from build123d import *

# Parameters (mm, degrees)
F1_DEPTH    = 12.7
F6_DEPTH    = 25.4
F7_T1_DEPTH = 49.4232912098
F7_T4_ANGLE = 29.8619681209
F7_T6_ANGLE = 29.8619681209
F8_START    = -2.159
F8_DEPTH    = 23.241
F9_DEPTH    = 25.4


# Not quite as in the source:
# - a fillet or chamfer that OpenCascade refuses, or shapes differently, is made with other operations: its cross-section is extruded or revolved along the edge and cut away or added


with BuildPart() as f1:
    # F0 (on Top) → F1 (new body, symmetric)
    with BuildSketch(Plane.XY):
        with BuildLine():
            ThreePointArc((0, 101.6), (-6.6449579298, 101.382466601), (-13.2614611296, 100.7307979156))
            Line((-13.2614611296, 100.7307979156), (-12.6812722051, 96.3238255068))
            ThreePointArc((-12.6812722051, 96.3238255068), (-6.3542410204, 96.9469836872), (0, 97.155))
            Line((0, 97.155), (0, 101.6))
        make_face()
        with BuildLine():
            Line((12.6812722051, 96.3238255068), (13.2614611296, 100.7307979156))
            ThreePointArc((13.2614611296, 100.7307979156), (6.6449579298, 101.382466601), (0, 101.6))
            Line((0, 101.6), (0, 97.155))
            ThreePointArc((0, 97.155), (6.3542410204, 96.9469836872), (12.6812722051, 96.3238255068))
        make_face()
    extrude(amount=F1_DEPTH, both=True)

    # F5 (on line) → F6 (cut)
    with BuildSketch(Plane(origin=(0, 101.6, 0), x_dir=(-1, 0, 0), z_dir=(0, 1, 0))):
        with BuildLine():
            Line((6.35, -6.35), (4.9276, -6.35))
            ThreePointArc((4.9276, -6.35), (6.35, -7.7724), (7.7724, -6.35))
            ThreePointArc((7.7724, -6.35), (7.3557886856, -5.3442113144), (6.35, -4.9276))
            Line((6.35, -4.9276), (6.35, -6.35))
        make_face()
        with BuildLine():
            ThreePointArc((6.35, -4.9276), (5.3442113144, -5.3442113144), (4.9276, -6.35))
            Line((4.9276, -6.35), (6.35, -6.35))
            Line((6.35, -6.35), (6.35, -4.9276))
        make_face()
        with BuildLine():
            Line((-4.9276, -6.35), (-6.35, -6.35))
            Line((-6.35, -6.35), (-6.35, -4.9276))
            ThreePointArc((-6.35, -4.9276), (-7.3557886856, -7.3557886856), (-4.9276, -6.35))
        make_face()
        with BuildLine():
            Line((-6.35, -4.9276), (-6.35, -6.35))
            Line((-6.35, -6.35), (-4.9276, -6.35))
            ThreePointArc((-4.9276, -6.35), (-5.3442113144, -5.3442113144), (-6.35, -4.9276))
        make_face()
        with BuildLine():
            Line((6.35, 6.35), (6.35, 4.9276))
            ThreePointArc((6.35, 4.9276), (7.3557886856, 5.3442113144), (7.7724, 6.35))
            ThreePointArc((7.7724, 6.35), (6.35, 7.7724), (4.9276, 6.35))
            Line((4.9276, 6.35), (6.35, 6.35))
        make_face()
        with BuildLine():
            ThreePointArc((4.9276, 6.35), (5.3442113144, 5.3442113144), (6.35, 4.9276))
            Line((6.35, 4.9276), (6.35, 6.35))
            Line((6.35, 6.35), (4.9276, 6.35))
        make_face()
        with BuildLine():
            ThreePointArc((-4.9276, 6.35), (-7.3557886856, 7.3557886856), (-6.35, 4.9276))
            Line((-6.35, 4.9276), (-6.35, 6.35))
            Line((-6.35, 6.35), (-4.9276, 6.35))
        make_face()
        with BuildLine():
            Line((-6.35, 6.35), (-6.35, 4.9276))
            ThreePointArc((-6.35, 4.9276), (-5.3442113144, 5.3442113144), (-4.9276, 6.35))
            Line((-4.9276, 6.35), (-6.35, 6.35))
        make_face()
    extrude(amount=-F6_DEPTH, mode=Mode.SUBTRACT)

    # F7: fillet of radius 5.08 on 4 edges, made by hand

    # F7_s2 → F7_t1 (cut)
    with BuildSketch(Plane.XY.offset(-24.7116456049)):
        with BuildLine():
            ThreePointArc((7.9036679621, 96.8329802172), (11.3054660928, 97.7882158705), (13.2614611296, 100.7307979156))
            Line((13.2614611296, 100.7307979156), (12.6812722051, 96.3238255068))
            ThreePointArc((12.6812722051, 96.3238255068), (10.2956180024, 96.6079410553), (7.9036679621, 96.8329802172))
        make_face()
        with BuildLine():
            ThreePointArc((-7.9036679621, 96.8329802172), (-11.3054660928, 97.7882158705), (-13.2614611296, 100.7307979156))
            Line((-13.2614611296, 100.7307979156), (-12.6812722051, 96.3238255068))
            ThreePointArc((-12.6812722051, 96.3238255068), (-10.2956180024, 96.6079410553), (-7.9036679621, 96.8329802172))
        make_face()
    extrude(amount=F7_T1_DEPTH, mode=Mode.SUBTRACT)

    # F7_s3 → F7_t4 (revolve, cut)
    with BuildSketch(Plane(origin=(0, 0, 0), x_dir=(0, 0, 1), z_dir=(-0.9662368873, -0.2576553465, 0))):
        with BuildLine():
            ThreePointArc((7.6598437524, 97.155), (11.0199479175, 98.425), (12.7, 101.6))
            Line((12.7, 101.6), (12.7, 97.155))
            Line((12.7, 97.155), (7.6598437524, 97.155))
        make_face()
    revolve(axis=Axis((0, 0, 12.7), (0, 0, -1)), revolution_arc=F7_T4_ANGLE, mode=Mode.SUBTRACT)

    # F7_s5 → F7_t6 (revolve, cut)
    with BuildSketch(Plane(origin=(0, 0, 0), x_dir=(0, 0, 1), z_dir=(-0.9662368873, -0.2576553465, 0))):
        with BuildLine():
            ThreePointArc((-7.6598437524, 97.155), (-11.0199479175, 98.425), (-12.7, 101.6))
            Line((-12.7, 101.6), (-12.7, 97.155))
            Line((-12.7, 97.155), (-7.6598437524, 97.155))
        make_face()
    revolve(axis=Axis((0, 0, -12.7), (0, 0, -1)), revolution_arc=F7_T6_ANGLE, mode=Mode.SUBTRACT)

    # F5 (on line) → F8 (cut)
    with BuildSketch(Plane(origin=(0, 101.6, 0), x_dir=(-1, 0, 0), z_dir=(0, 1, 0)).offset(F8_START)):
        with BuildLine():
            Line((6.35, 4.9276), (6.35, 2.6838257906))
            Line((6.35, 2.6838257906), (9.525, 4.5169128953))
            Line((9.525, 4.5169128953), (9.525, 8.1830871047))
            Line((9.525, 8.1830871047), (6.35, 10.0161742094))
            Line((6.35, 10.0161742094), (3.175, 8.1830871047))
            Line((3.175, 8.1830871047), (3.175, 6.35))
            Line((3.175, 6.35), (4.9276, 6.35))
            ThreePointArc((4.9276, 6.35), (6.35, 7.7724), (7.7724, 6.35))
            ThreePointArc((7.7724, 6.35), (7.3557886856, 5.3442113144), (6.35, 4.9276))
        make_face()
        with BuildLine():
            Line((3.175, 4.5169128953), (6.35, 2.6838257906))
            Line((6.35, 2.6838257906), (6.35, 4.9276))
            ThreePointArc((6.35, 4.9276), (5.3442113144, 5.3442113144), (4.9276, 6.35))
            Line((4.9276, 6.35), (3.175, 6.35))
            Line((3.175, 6.35), (3.175, 4.5169128953))
        make_face()
        with BuildLine():
            Line((4.9276, -6.35), (3.175, -6.35))
            Line((3.175, -6.35), (3.175, -8.1830871047))
            Line((3.175, -8.1830871047), (6.35, -10.0161742094))
            Line((6.35, -10.0161742094), (9.525, -8.1830871047))
            Line((9.525, -8.1830871047), (9.525, -4.5169128953))
            Line((9.525, -4.5169128953), (6.35, -2.6838257906))
            Line((6.35, -2.6838257906), (6.35, -4.9276))
            ThreePointArc((6.35, -4.9276), (7.3557886856, -5.3442113144), (7.7724, -6.35))
            ThreePointArc((7.7724, -6.35), (6.35, -7.7724), (4.9276, -6.35))
        make_face()
        with BuildLine():
            Line((3.175, -4.5169128953), (3.175, -6.35))
            Line((3.175, -6.35), (4.9276, -6.35))
            ThreePointArc((4.9276, -6.35), (5.3442113144, -5.3442113144), (6.35, -4.9276))
            Line((6.35, -4.9276), (6.35, -2.6838257906))
            Line((6.35, -2.6838257906), (3.175, -4.5169128953))
        make_face()
        with BuildLine():
            Line((-3.175, -6.35), (-4.9276, -6.35))
            ThreePointArc((-4.9276, -6.35), (-7.3557886856, -7.3557886856), (-6.35, -4.9276))
            Line((-6.35, -4.9276), (-6.35, -2.6838257906))
            Line((-6.35, -2.6838257906), (-9.525, -4.5169128953))
            Line((-9.525, -4.5169128953), (-9.525, -8.1830871047))
            Line((-9.525, -8.1830871047), (-6.35, -10.0161742094))
            Line((-6.35, -10.0161742094), (-3.175, -8.1830871047))
            Line((-3.175, -8.1830871047), (-3.175, -6.35))
        make_face()
        with BuildLine():
            ThreePointArc((-6.35, -4.9276), (-5.3442113144, -5.3442113144), (-4.9276, -6.35))
            Line((-4.9276, -6.35), (-3.175, -6.35))
            Line((-3.175, -6.35), (-3.175, -4.5169128953))
            Line((-3.175, -4.5169128953), (-6.35, -2.6838257906))
            Line((-6.35, -2.6838257906), (-6.35, -4.9276))
        make_face()
        with BuildLine():
            Line((-6.35, 4.9276), (-6.35, 2.6838257906))
            Line((-6.35, 2.6838257906), (-3.175, 4.5169128953))
            Line((-3.175, 4.5169128953), (-3.175, 6.35))
            Line((-3.175, 6.35), (-4.9276, 6.35))
            ThreePointArc((-4.9276, 6.35), (-5.3442113144, 5.3442113144), (-6.35, 4.9276))
        make_face()
        with BuildLine():
            Line((-9.525, 4.5169128953), (-6.35, 2.6838257906))
            Line((-6.35, 2.6838257906), (-6.35, 4.9276))
            ThreePointArc((-6.35, 4.9276), (-7.3557886856, 7.3557886856), (-4.9276, 6.35))
            Line((-4.9276, 6.35), (-3.175, 6.35))
            Line((-3.175, 6.35), (-3.175, 8.1830871047))
            Line((-3.175, 8.1830871047), (-6.35, 10.0161742094))
            Line((-6.35, 10.0161742094), (-9.525, 8.1830871047))
            Line((-9.525, 8.1830871047), (-9.525, 4.5169128953))
        make_face()
    extrude(amount=-F8_DEPTH, mode=Mode.SUBTRACT)

    # F5 (on line) → F9 (cut)
    with BuildSketch(Plane(origin=(0, 101.6, 0), x_dir=(-1, 0, 0), z_dir=(0, 1, 0))):
        with BuildLine():
            ThreePointArc((-4.9276, 6.35), (-7.3557886856, 7.3557886856), (-6.35, 4.9276))
            Line((-6.35, 4.9276), (-6.35, 6.35))
            Line((-6.35, 6.35), (-4.9276, 6.35))
        make_face()
        with BuildLine():
            Line((-6.35, 6.35), (-6.35, 4.9276))
            ThreePointArc((-6.35, 4.9276), (-5.3442113144, 5.3442113144), (-4.9276, 6.35))
            Line((-4.9276, 6.35), (-6.35, 6.35))
        make_face()
    extrude(amount=-F9_DEPTH, mode=Mode.SUBTRACT)


solid = f1.part
Read the model definition and answer for the solid it produces. Units are mm, in the model's axes. A direction names the side the tool comes from. Round coordinates to 2 decimals unless told otherwise and drop trailing zeros. Write each loop counter-clockwise with the first axis right and the second up, starting at its lowest first coordinate (ties: lowest second). Pieces come first, ordered by that corner, then holes. Notation, with made-up numbers: (5, 33) - (63, 33) arc R25 ccw to (63, 47) - close; hole circle Ø8 at (57, 73). An arc over 180 degrees is marked (long way). Use a Markdown table: item, result.
(1) Each of these flat-tipped pins is pushed along its axis until it touches: pin 1 Ø2.5 at (y, z) = (97.5, -5.5) entering from +X; pin 2 Ø2 at (y, z) = (98.5, -4) entering from +X; pin 3 Ø2.5 at (y, z) = (98, 5.5) entering from -X; pin 4 Ø2.5 at (x, z) = (6.35, -6.35) entering from -Y. Where does it stop, or does it pass through?
Reported:
| item | result |
|---|---|
| pin 1 | x = 12.31 |
| pin 2 | x = 12.8 |
| pin 3 | x = -12.65 |
| pin 4 | through |
(2) The mould has two halves that part along X. Classify faces 3 (the flat face through (7.96, 98.159, -9.087)), 4 (the flat face through (9.525, 98, -6)): released by +X, released by -X, zero draft, split by the parting line, or undercut.
Reported:
| item | result |
|---|---|
| face 3 | undercut |
| face 4 | undercut |
(3) The part is cut by section B-B (y = 98.95). State how many separate pieces and enclosed holes the cut face has, then the cut area to 3 significant figures.
Reported:
| item | result |
|---|---|
| separate pieces | 1 |
| enclosed holes | 4 |
| area | 445 mm2 |
(4) Which of the six approach directions +Z, -Z, +X, -X, +Y, -Y give full straight-line access (tool end or side, diameter ignored) to faces 1 (the flat face through (4.78, 98.21, 3.59)), 2 (the cylindrical face through (-0.111, 97.155, 0.107))?
Reported:
| item | result |
|---|---|
| face 1 | -Y |
| face 2 | +Z, -Z, -Y |
(5) Straight lines are drawn through the part: line 1 along Z through (x, y) = (-8.5, 98.8); line 2 along Z through (x, y) = (3.5, 97.6); line 3 along X through (y, z) = (100.55, -6.35). For each, find the intervals that lie inside material, in ascending order. Write a range as [from, to].
Reported:
| item | result |
|---|---|
| line 1 | [-11.71, -8.77], [-3.93, 3.93], [8.77, 11.71] |
| line 2 | [-9.87, -8.37], [-4.33, 4.33], [8.37, 9.87] |
| line 3 | [-13.22, -7.77], [-4.93, 4.93], [7.77, 13.22] |
(6) The part is cut by section A-A (z = 3). Write down the section's boundary in (x, y) (3 decimals), then the cut area to 3 significant figures.
Reported:
| item | result |
|---|---|
| outline | (-13.261, 100.731) arc R5.08 ccw to (-7.904, 96.833) arc R97.155 cw to (-6.898, 96.91) - (-6.898, 99.441) - (-5.802, 99.441) - (-5.802, 96.982) arc R97.155 cw to (5.802, 96.982) - (5.802, 99.441) - (6.898, 99.441) - (6.898, 96.91) arc R97.155 cw to (7.904, 96.833) arc R5.08 ccw to (13.261, 100.731) arc R101.6 ccw to start |
| area | 100 mm2 |
